Study the drawing (mm; zero at the part's minimum x, y, z) and answer. A direction names the side the tool comes from. Coordinates: 2 decimals unless noted, no trailing zeros. Loops run counter-clockwise (first coordinate to the right, second up) from the corner with the lowest first, then second, coordinate; pieces in that order, holes last.
Q1. Section B-B (y = 14.75) is taken. Give the vertices of the cut face in (x, z), then the cut area to 3 significant figures.
Q2. Section C-C (z = 1) is taken. Give the vertices of the cut face in (x, y).
Q3. Section A-A (z = 5) is taken. Give the vertices of the cut face in (x, y), then the cut area to 3 significant figures.
Q4. Flat-ended cylindrical pins translate along their axes: P1, Ø2, axis at y = 3, z = 4, coming from the -X side; P2, Ø5, axis at x = 7.5, z = 2, coming from the -Y side; P3, Ø3.5, axis at y = 11.5, z = 2.5, coming from the +X side. Find the tip coordinate at first contact, or state that the pin passes through.
Q5. Section D-D (x = 12.75) is taken. Give the vertices of the cut face in (y, z).
Q6. The mould has two halves that part along Z. Classify the marked faces 4, 5 and 6: pulls with the +Z half, pulls with the -Z half, needs draft (parallel to the pull), parting line crosses it, or undercut.
Q7. Straight lines are drawn through the part: line 1 (Y direction, x = 0.6, z = 5); line 2 (X direction, y = 5.5, z = 9); line 3 (Y direction, x = 8.5, z = 9.25). For each, find the intervals that lie inside material, in ascending order.
Q8. Which of the six approach directions +Z, -Z, +X, -X, +Y, -Y give full straight-line access (tool end or side, diameter ignored) to the marked faces 1, 2 and 3?
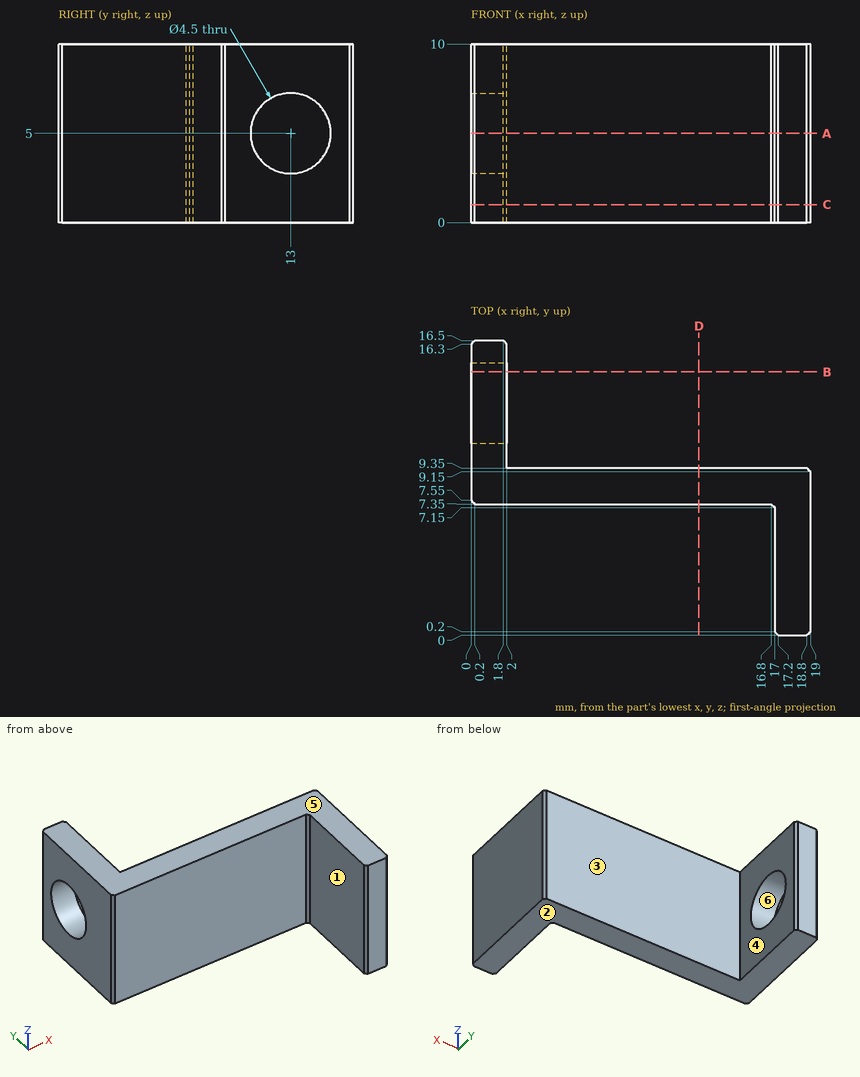
Numbers:
1. outline: (0, 0) - (2, 0) - (2, 3.59) - (0, 3.59) - close; (0, 6.41) - (2, 6.41) - (2, 10) - (0, 10) - close
1. area: 14.3 mm2
2. outline: (0, 7.55) - (0.2, 7.35) - (16.8, 7.35) - (17, 7.15) - (17, 0.2) - (17.2, 0) - (18.8, 0) - (19, 0.2) - (19, 9.15) - (18.8, 9.35) - (2, 9.35) - (2, 16.3) - (1.8, 16.5) - (0.2, 16.5) - (0, 16.3) - close
3. outline: (0, 7.55) - (0.2, 7.35) - (16.8, 7.35) - (17, 7.15) - (17, 0.2) - (17.2, 0) - (18.8, 0) - (19, 0.2) - (19, 9.15) - (18.8, 9.35) - (2, 9.35) - (2, 10.75) - (0, 10.75) - close; (0, 15.25) - (2, 15.25) - (2, 16.3) - (1.8, 16.5) - (0.2, 16.5) - (0, 16.3) - close
3. area: 57.9 mm2
4. P1: stops at x = 17
4. P2: stops at y = 7.35
4. P3: stops at x = 2
5. outline: (7.35, 0) - (9.35, 0) - (9.35, 10) - (7.35, 10) - close
6. face 4: needs draft
6. face 5: pulls with the +Z half
6. face 6: undercut
7. line 1: y = 7.35 to 10.75, 15.25 to 16.5
7. line 2: x = 17 to 19
7. line 3: y = 7.35 to 9.35
8. face 1: +Z, -Z, -X, -Y
8. face 2: -Z, +X, -X, +Y, -Y
8. face 3: +Z, -Z, +X, +Y
